Geometry check sheet. Reference: the model listing, model coordinates, mm. Face numbers are marked on the shaded views. A direction names the side the tool comes from. Give positions to 0.01 mm unless a question says otherwise; leave off trailing zeros. Loops run counter-clockwise (first coordinate to the right, second up) from the corner with the lowest first, then second, coordinate; pieces in that order, holes last. Notation, with made-up numbers: (15, 6.25) - (51, 6.25) arc R37 ccw to (51, 44.25) - close; hole circle Ø11 at (50.25, 72). An arc over 180 degrees is marked (long way). One line per question, with ' | ' between items. Start each with the question number.
from build123d import *

# Parameters (mm, degrees)
F0_W           = 30
F0_H           = 30
F1_DEPTH       = 30
F3_D           = 9
F3_CBORE_D     = 14.25
F3_CBORE_DEPTH = 27
F5_D           = 9
F5_CBORE_D     = 14.25
F5_CBORE_DEPTH = 27
F7_D           = 9
F7_CBORE_D     = 14.25
F7_CBORE_DEPTH = 27


with BuildPart() as f1:
    # F0 (on Front) → F1 (new body)
    with BuildSketch(Plane.XZ):
        Rectangle(F0_W, F0_H)
    extrude(amount=F1_DEPTH)

    # F3 (through all)
    with Locations(Plane.XZ.offset(30)):
        with Locations((0, 0)):
            CounterBoreHole(F3_D / 2, F3_CBORE_D / 2, F3_CBORE_DEPTH)

    # F5 (through all)
    with Locations(Plane(origin=(-15, 0, 0), x_dir=(0, -1, 0), z_dir=(-1, 0, 0))):
        with Locations((15, 0)):
            CounterBoreHole(F5_D / 2, F5_CBORE_D / 2, F5_CBORE_DEPTH)

    # F7 (through all)
    with Locations(Plane(origin=(0, 0, -15), x_dir=(1, 0, 0), z_dir=(0, 0, -1))):
        with Locations((0, 15)):
            CounterBoreHole(F7_D / 2, F7_CBORE_D / 2, F7_CBORE_DEPTH)


solid = f1.part
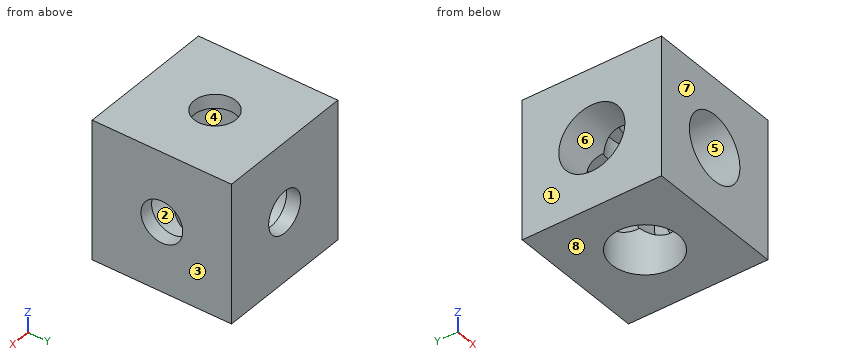
(1) Section check B-B, the plane z = 0. Record the boundary of the cut face in (x, y) (3 decimals).
(2) Section check C-C, the plane y = -21.5. Record the boundary of the cut face in (x, z) (3 decimals).
(3) Material ranges on line 1 (Y direction, x = 0, z = 12.7); line 2 (Y direction, x = 0, z = -10.5) (3 decimals); line 3 (Z direction, x = 14.1, y = -15), recorded low to high.
(4) Mould release check, pull along Z, two halves, no side actions. Record for the marked faces 6, 7 and 8: pulls with the +Z half, pulls with the -Z half, needs draft (parallel to the pull), parting line crosses it, or undercut.
(5) Section check D-D, the plane z = 13.25. Record the boundary of the cut face in (x, y).
(6) Depth check by flat-ended pin: pin 1 Ø4.5 at (x, z) = (-3, -2) entering from -Y; pin 2 Ø10.5 at (x, y) = (0, -15) entering from -Z; pin 3 Ø5.5 at (x, z) = (0, 0) entering from +Y; pin 4 Ø4.5 at (y, z) = (-12.5, 1) entering from -X. Enter the tip coordinate at first touch or a pass-through.
(7) Section check A-A, the plane x = 0. Record the boundary of the cut face in (y, z) (3 decimals), and give its area (3 significant figures).
(8) Tool access check on the marked faces 1, 2, 3, 4 and 5. Record the directions out of +Z, -Z, +X, -X, +Y, -Y that give a thin tool (end or side, any length) a straight path to the whole face; none if there is none.
Numbers:
1) outline: (-15, -30) - (-7.125, -30) - (-7.125, -22.125) - (-15, -22.125) - close; (-15, -7.875) - (-7.125, -7.875) - (-7.125, -3) - (-4.5, -3) - (-4.5, 0) - (-15, 0) - close; (4.5, -3) - (7.125, -3) - (7.125, -7.875) - (12, -7.875) - (12, -10.5) - (15, -10.5) - (15, 0) - (4.5, 0) - close; (7.125, -30) - (15, -30) - (15, -19.5) - (12, -19.5) - (12, -22.125) - (7.125, -22.125) - close
2) outline: (-15, -15) - (-2.918, -15) - (-2.918, -6.5) arc R7.125 cw to (-6.5, -2.918) - (-15, -2.918) - close; (-15, 2.918) - (-6.5, 2.918) arc R7.125 cw to (-2.918, 6.5) - (-2.918, 12) - (2.918, 12) - (2.918, 6.5) arc R7.125 cw to (6.5, 2.918) - (12, 2.918) - (12, -2.918) - (6.5, -2.918) arc R7.125 cw to (2.918, -6.5) - (2.918, -15) - (15, -15) - (15, 15) - (-15, 15) - close
3) line 1: -30 to -19.5, -10.5 to 0 | line 2: -30 to -22.125, -7.875 to 0 | line 3: -15 to -4.5, 4.5 to 15
4) face 6: undercut | face 7: needs draft | face 8: pulls with the -Z half
5) outline: (-15, -30) - (15, -30) - (15, 0) - (-15, 0) - close; hole circle Ø9 at (0, -15)
6) pin 1: y = -3 | pin 2: z = 12 | pin 3: through | pin 4: x = 12
7) outline: (-30, -15) - (-22.125, -15) - (-22.125, -7.125) - (-30, -7.125) - close; (-30, 7.125) - (-22.125, 7.125) - (-22.125, 12) - (-19.5, 12) - (-19.5, 15) - (-30, 15) - close; (-10.5, 12) - (-7.875, 12) - (-7.875, 7.125) - (-3, 7.125) - (-3, 4.5) - (0, 4.5) - (0, 15) - (-10.5, 15) - close; (-7.875, -15) - (0, -15) - (0, -4.5) - (-3, -4.5) - (-3, -7.125) - (-7.875, -7.125) - close | area: 280 mm^2
8) face 1: +Z, -Z, -X, +Y, -Y | face 2: -X | face 3: +Z, -Z, +X, +Y, -Y | face 4: -Z | face 5: -Y
